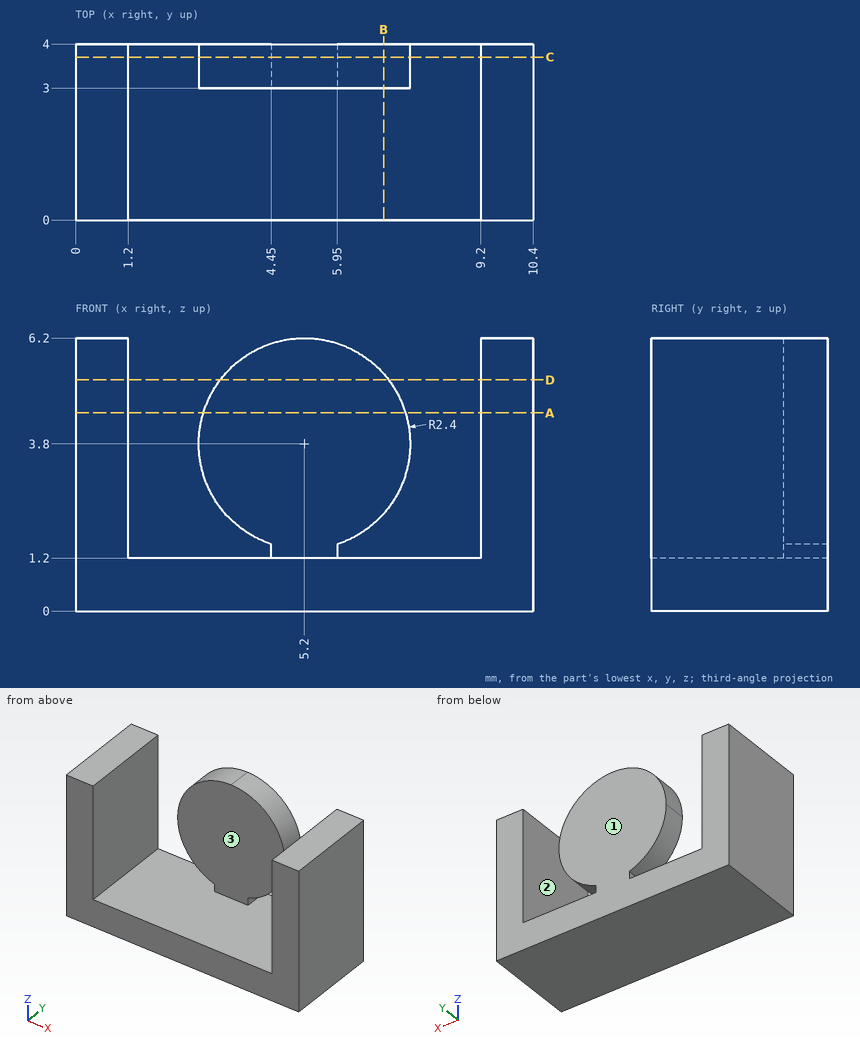
Input: dimensioned drawing with shaded views. Units: mm. Origin: part minimum x, y, z. A direction names the side the tool comes from. Coordinates: 2 decimals unless noted, no trailing zeros. Order: outer loops, then holes, each group sorted by start corner. A loop starts at its lowest first (then second) coordinate and runs counter-clockwise, first axis right, second up. Notation, with made-up numbers: M -21,8 L 37,8 A17 ccw 37,30 Z; hole C 35,48 d9. An arc over 180 degrees is marked long. Write each question's results on one line, items separated by ' | '. Start each with the question number.
Item 1: First-contact query: pin 1 Ø2 at (x, y) = (7, 1.5) entering from +Z. Flat tip, straight axial feed; report the tip coordinate or a pass-through.
Item 2: Set-up query: the marked faces 1, 2 and 3. Return all of +Z, -Z, +X, -X, +Y, -Y with unobstructed straight access to the full face (end or side cutting, diameter ignored); none if empty.
Item 3: Cut plane A-A (z = 4.5). Return loops of the section in (x, y).
Item 4: Cut plane C-C (y = 3.7). Return loops of the section in (x, z), and give its area (3 significant figures).
Item 5: Cut plane D-D (z = 5.25). Return loops of the section in (x, y), and give its area (3 significant figures).
Item 6: Cut plane B-B (x = 7). Return loops of the section in (y, z).
Item 7: Line query: probe 1 along X at (y, z) = (2.35, 5.75); probe 2 along X at (y, z) = (3.35, 2.5); probe 3 along Z at (x, y) = (6.75, 1.85). Output: solid intervals per line, ascending.
Checked values:
1) pin 1: stops at z = 1.2
2) face 1: +Z, -Z, +X, -X, +Y | face 2: +Z, +Y, -Y | face 3: +Z, -Y
3) outline: M 0,0 L 1.2,0 L 1.2,4 L 0,4 Z; M 2.9,3 L 7.5,3 L 7.5,4 L 2.9,4 Z; M 9.2,0 L 10.4,0 L 10.4,4 L 9.2,4 Z
4) outline: M 0,0 L 10.4,0 L 10.4,6.2 L 9.2,6.2 L 9.2,1.2 L 5.95,1.2 L 5.95,1.52 A2.4 ccw long 4.45,1.52 L 4.45,1.2 L 1.2,1.2 L 1.2,6.2 L 0,6.2 Z | area: 42.9 mm2
5) outline: M 0,0 L 1.2,0 L 1.2,4 L 0,4 Z; M 3.29,3 L 7.11,3 L 7.11,4 L 3.29,4 Z; M 9.2,0 L 10.4,0 L 10.4,4 L 9.2,4 Z | area: 13.4 mm2
6) outline: M 0,0 L 4,0 L 4,1.2 L 0,1.2 Z; M 3,2.21 L 4,2.21 L 4,5.39 L 3,5.39 Z
7) probe 1: x = 0 to 1.2, 9.2 to 10.4 | probe 2: x = 0 to 1.2, 3.18 to 7.22, 9.2 to 10.4 | probe 3: z = 0 to 1.2
